Part print with two shaded views. Sizes in mm from the minimum x, y, z corner. A direction names the side the tool comes from. Coordinates: 2 decimals unless noted, no trailing zeros. Order: outer loops, then holes, each group sorted by start corner. A loop starts at its lowest first (then second) coordinate and runs counter-clockwise, first axis right, second up. Notation, with made-up numbers: (-2, -31) - (43, -31) arc R26 ccw to (43, -12) - close; hole circle Ø8 at (67, -19). An arc over 180 degrees is marked (long way). One line per item, written item: value.
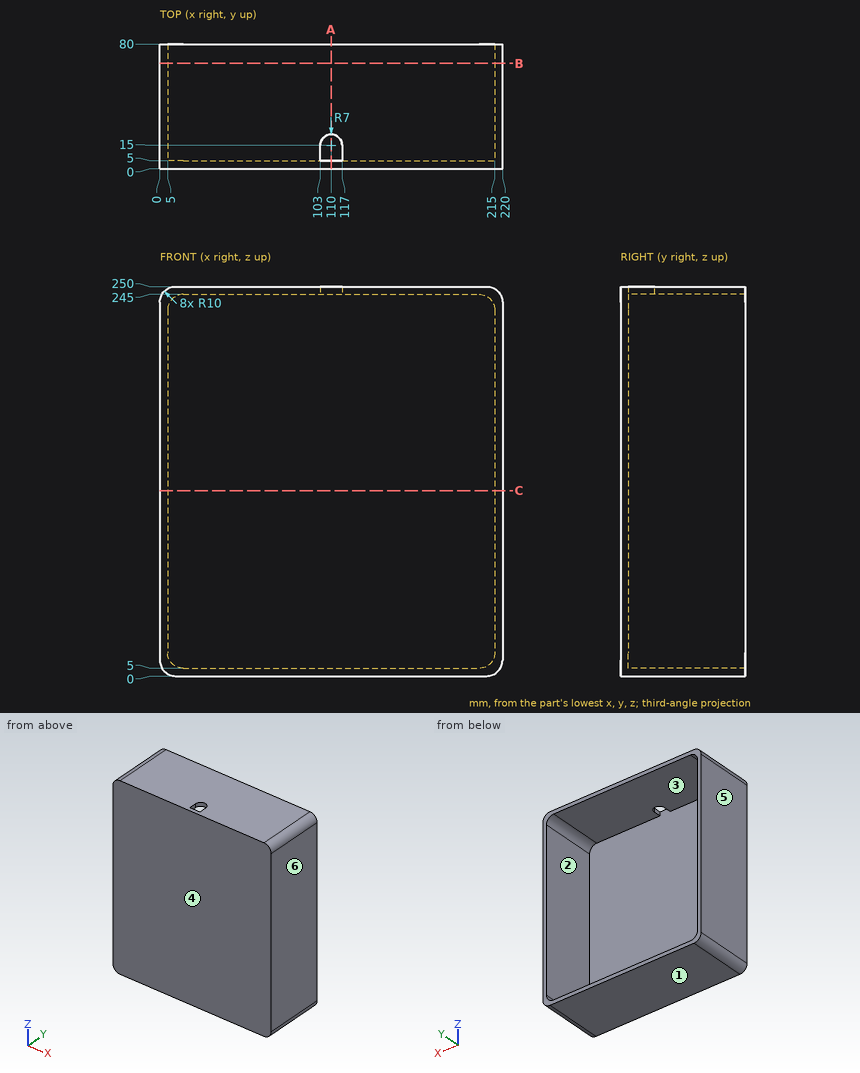
1. Two-plate mould, pull along X, no slides. Class the marked faces 3, 4, 5 and 6: pulls with the +X half, pulls with the -X half, needs draft (parallel to the pull), parting line crosses it, or undercut.
Values found:
face 3: undercut
face 4: needs draft
face 5: pulls with the -X half
face 6: pulls with the +X half
2. 3-axis set-ups, long thin cutter, end or side, ignore diameter. For the marked faces 1 and 2: which of +Z, -Z, +X, -X, +Y, -Y reach the whole face in a straight line?
Values found:
face 1: -Z, +X, -X, +Y, -Y
face 2: +Y
3. Band-saw the part on C-C, the plane z = 119. Give the cut face in (x, y), and give its area (3 significant figures).
Values found:
outline: (0, 0) - (220, 0) - (220, 80) - (215, 80) - (215, 5) - (5, 5) - (5, 80) - (0, 80) - close
area: 1,850 mm2
4. Band-saw the part on A-A, the plane x = 110. Give the cut face in (y, z), and give its area (4 significant figures).
Values found:
outline: (0, 0) - (80, 0) - (80, 5) - (5, 5) - (5, 250) - (0, 250) - close; (22, 245) - (80, 245) - (80, 250) - (22, 250) - close
area: 1,915 mm2
5. Probe line 1 along Z through (x, y) = (156.5, 20); line 2 along X through (y, z) = (55.5, 134); line 3 along Y through (x, z) = (110, 84). List the from-to ranges inside material, lowest first.
Values found:
line 1: z = 0 to 5, 245 to 250
line 2: x = 0 to 5, 215 to 220
line 3: y = 0 to 5
6. Flat gauge pins, fed straight in: P1, Ø5.5, axis at y = 9, z = 247, coming from the -X side; P2, Ø5.5, axis at y = 12, z = 248, coming from the +X side; P3, Ø4, axis at x = 112, z = 200, coming from the -Y side. Where does each tip first touch, or does it go through?
Values found:
P1: stops at x = 0.95
P2: stops at x = 218.51
P3: stops at y = 0
7. Band-saw the part on B-B, the plane y = 67.5. Give the cut face in (x, z), and give its area (3 significant figures).
Values found:
outline: (0, 10) arc R10 ccw to (10, 0) - (210, 0) arc R10 ccw to (220, 10) - (220, 240) arc R10 ccw to (210, 250) - (10, 250) arc R10 ccw to (0, 240) - close; hole (5, 15) arc R10 ccw to (15, 5) - (205, 5) arc R10 ccw to (215, 15) - (215, 235) arc R10 ccw to (205, 245) - (15, 245) arc R10 ccw to (5, 235) - close
area: 4,600 mm2
